```python
from build123d import *

# Parameters (mm, degrees)
FILLET1_R      = 0.3
CHAMFER1_SIZE  = 0.8
CHAMFER1_SIZE2 = 0.461880215
CHAMFER2_SIZE  = 0.5
CHAMFER2_SIZE2 = 0.288675135


with BuildPart() as part:
    # Sketch1 → Revolve1 (revolve)
    with BuildSketch(Plane.XY):
        Polygon((2.85, 0), (4.9, 0), (4.9, -1), (3.5, -1), (3.5, -12.9), (2.5, -12.9), (2.5, -5.7), (2.85, -5.7), align=None)
    revolve(axis=Axis((0, 0, 0), (0, -1, 0)))

    # Fillet1
    fillet1_edges = [part.edges().sort_by_distance(p)[0] for p in [
        (-4.9, -1, 0),
        (-4.9, 0, 0),
        (-2.85, 0, 0),
    ]]
    fillet(fillet1_edges, radius=FILLET1_R)

    # Chamfer1
    chamfer1_edges = [part.edges().sort_by_distance(p)[0] for p in [
        (-3.5, -12.9, 0),
    ]]
    chamfer1_side = [part.faces().sort_by_distance(p)[0] for p in [
        (-3.5, -6.95, 0),
    ]]
    chamfer(chamfer1_edges, length=CHAMFER1_SIZE, length2=CHAMFER1_SIZE2, reference=chamfer1_side[0])

    # Chamfer2
    chamfer2_edges = [part.edges().sort_by_distance(p)[0] for p in [
        (-2.5, -12.9, 0),
    ]]
    chamfer2_side = [part.faces().sort_by_distance(p)[0] for p in [
        (-2.5, -9.3, 0),
    ]]
    chamfer(chamfer2_edges, length=CHAMFER2_SIZE, length2=CHAMFER2_SIZE2, reference=chamfer2_side[0])


solid = part.part
```
Verification items for the finished model (mm, model axes). A direction names the side the tool comes from. Give positions to 0.01 mm unless a question says otherwise; leave off trailing zeros. Order: outer loops, then holes, each group sorted by start corner. A loop starts at its lowest first (then second) coordinate and runs counter-clockwise, first axis right, second up. Notation, with made-up numbers: (-9, 24) -> (29, 24) arc R19 cw to (29, 45) -> close; hole circle Ø9 at (69, 4.5). An arc over 180 degrees is marked (long way). Use a Markdown table: item, result.
1) Section check D-D, the plane y = -10.25. Record the boundary of the cut face in (x, z), then the cut area to 3 significant figures.
Results:
| item | result |
|---|---|
| outline | circle Ø7 at (0, 0); hole circle Ø5 at (0, 0) |
| area | 18.8 mm² |
2) Section check B-B, the plane x = 0. Record the boundary of the cut face in (y, z).
Results:
| item | result |
|---|---|
| outline | (-12.9, -3.04) -> (-12.1, -3.5) -> (-1, -3.5) -> (-1, -4.6) arc R0.3 ccw to (-0.7, -4.9) -> (-0.3, -4.9) arc R0.3 ccw to (0, -4.6) -> (0, -3.15) arc R0.3 ccw to (-0.3, -2.85) -> (-5.7, -2.85) -> (-5.7, -2.5) -> (-12.4, -2.5) -> (-12.9, -2.79) -> close; (-12.9, 2.79) -> (-12.4, 2.5) -> (-5.7, 2.5) -> (-5.7, 2.85) -> (-0.3, 2.85) arc R0.3 ccw to (0, 3.15) -> (0, 4.6) arc R0.3 ccw to (-0.3, 4.9) -> (-0.7, 4.9) arc R0.3 ccw to (-1, 4.6) -> (-1, 3.5) -> (-12.1, 3.5) -> (-12.9, 3.04) -> close |
3) Section check A-A, the plane z = 0. Record the boundary of the cut face in (x, y).
Results:
| item | result |
|---|---|
| outline | (-4.9, -0.7) arc R0.3 ccw to (-4.6, -1) -> (-3.5, -1) -> (-3.5, -12.1) -> (-3.04, -12.9) -> (-2.79, -12.9) -> (-2.5, -12.4) -> (-2.5, -5.7) -> (-2.85, -5.7) -> (-2.85, -0.3) arc R0.3 ccw to (-3.15, 0) -> (-4.6, 0) arc R0.3 ccw to (-4.9, -0.3) -> close; (2.5, -12.4) -> (2.79, -12.9) -> (3.04, -12.9) -> (3.5, -12.1) -> (3.5, -1) -> (4.6, -1) arc R0.3 ccw to (4.9, -0.7) -> (4.9, -0.3) arc R0.3 ccw to (4.6, 0) -> (3.15, 0) arc R0.3 ccw to (2.85, -0.3) -> (2.85, -5.7) -> (2.5, -5.7) -> close |
4) Material ranges on probe 1 along Z at (x, y) = (0, -1.35); probe 2 along Z at (x, y) = (0, -8); probe 3 along Y at (x, z) = (-3.25, 2.75), recorded low to high.
Results:
| item | result |
|---|---|
| probe 1 | -3.5 to -2.85, 2.85 to 3.5 |
| probe 2 | -3.5 to -2.5, 2.5 to 3.5 |
| probe 3 | -1 to 0 |
5) Mould release check, pull along Z, two halves, no side actions. Record for faces 1 (the cylindrical face through (-2.262, -2.962, -1.734)), 2 (the cylindrical face through (-1.062, -0.503, -4.783)), 3 (the flat face through (-2, 0, -3)): pulls with the +Z half, pulls with the -Z half, needs draft (parallel to the pull), parting line crosses it, or undercut.
Results:
| item | result |
|---|---|
| face 1 | undercut |
| face 2 | parting line crosses it |
| face 3 | needs draft |
6) Section check C-C, the plane y = -5.5. Record the boundary of the cut face in (x, z).
Results:
| item | result |
|---|---|
| outline | circle Ø7 at (0, 0); hole circle Ø5.7 at (0, 0) |
7) Depth check by flat-ended pin: pin 1 Ø1 at (x, y) = (-2.5, -7.5) entering from -Z; pin 2 Ø5 at (y, z) = (-9, 2.5) entering from +X; pin 3 Ø2 at (x, y) = (3, -10.5) entering from +Z; pin 4 Ø3.5 at (x, z) = (0, 0) entering from +Y (1 decimal). Enter the tip coordinate at first touch or a pass-through.
Results:
| item | result |
|---|---|
| pin 1 | z = -2.87 |
| pin 2 | x = 3.5 |
| pin 3 | z = 2.87 |
| pin 4 | through |
8) Tool access check on faces 4 (the cylindrical face through (-0.54, -9, -2.44)), 5 (the cylindrical face through (3.233, -6.628, -1.341)). Record the directions out of +Z, -Z, +X, -X, +Y, -Y that give a thin tool (end or side, any length) a straight path to the whole face; none if there is none.
Results:
| item | result |
|---|---|
| face 4 | +Y, -Y |
| face 5 | -Y |
